from build123d import *

# Parameters (mm, degrees)
SKETCH1_W           = 120
SKETCH1_H           = 35
BOSS_EXTRUDE1_DEPTH = 40
SKETCH2_W           = 21.39
SKETCH2_H           = 30
SKETCH2_W_2         = 22
SKETCH2_W_3         = 19.56
CUT_EXTRUDE1_DEPTH  = 30
SKETCH3_W           = 21.39
SKETCH3_H           = 22.392557851
SKETCH3_W_2         = 22
SKETCH3_W_3         = 19.56
SKETCH3_H_2         = 23.276606707
CUT_EXTRUDE2_DEPTH  = 8
FILLET1_R           = 10
SKETCH4_R           = 1.25
BOSS_EXTRUDE2_DEPTH = 4
BOSS_EXTRUDE3_DEPTH = 35


with BuildPart() as part:
    # Sketch1 → Boss-Extrude1 (new body)
    with BuildSketch(Plane(origin=(0, 0, 0), x_dir=(1, 0, 0), z_dir=(0, 1, 0))):
        with Locations((18.660377358, 10.962264151)):
            Rectangle(SKETCH1_W, SKETCH1_H)
    extrude(amount=BOSS_EXTRUDE1_DEPTH)

    # Sketch2 → Cut-Extrude1 (cut)
    with BuildSketch(Plane(origin=(0, 40, 0), x_dir=(1, 0, 0), z_dir=(0, 1, 0))):
        with Locations((-28.204622642, 8.462264151)):
            Rectangle(SKETCH2_W, SKETCH2_H)
        with Locations((-4.509622642, 8.462264151)):
            Rectangle(SKETCH2_W_2, SKETCH2_H)
        with Locations((19.490377358, 8.462264151)):
            Rectangle(SKETCH2_W_2, SKETCH2_H)
        with Locations((43.490377358, 8.462264151)):
            Rectangle(SKETCH2_W_2, SKETCH2_H)
        with Locations((66.270377358, 8.462264151)):
            Rectangle(SKETCH2_W_3, SKETCH2_H)
    extrude(amount=-CUT_EXTRUDE1_DEPTH, mode=Mode.SUBTRACT)

    # Sketch3 → Cut-Extrude2 (cut)
    with BuildSketch(Plane(origin=(0, 10, 0), x_dir=(1, 0, 0), z_dir=(0, 1, 0))):
        with Locations((-28.204622642, 12.265985226)):
            Rectangle(SKETCH3_W, SKETCH3_H)
        with Locations((-4.509622642, 12.265985226)):
            Rectangle(SKETCH3_W_2, SKETCH3_H)
        with Locations((19.490377358, 12.265985226)):
            Rectangle(SKETCH3_W_2, SKETCH3_H)
        with Locations((43.490377358, 12.265985226)):
            Rectangle(SKETCH3_W_2, SKETCH3_H)
        with Locations((66.270377358, 11.823960798)):
            Rectangle(SKETCH3_W_3, SKETCH3_H_2)
    extrude(amount=-CUT_EXTRUDE2_DEPTH, mode=Mode.SUBTRACT)

    # Fillet1
    # the kernel refuses this fillet: 10 mm, written as the material it adds along each edge
    with BuildSketch(Plane(origin=(76.050377358, 2, -0.185657444), x_dir=(0, 0, -1), z_dir=(-1, 0, 0))) as fillet1_piece_1:
        with BuildLine():
            CenterArc((9.797958971, -10), FILLET1_R, 90, 78.463040967)
            Line((0, -8), (-0.195959179, -7.96))
            ThreePointArc((-0.195959179, -7.96), (-0.2, -4), (-0.2, 0))
            Line((-0.2, 0), (0, 0.2))
            Line((0, 0.2), (9.797958971, 0.2))
            Line((9.797958971, 0.2), (9.797958971, 0))
        make_face()
    extrude(amount=44.054897428)
    with BuildSketch(Plane(origin=(54.490377358, 2, -1.0697063), x_dir=(0, 1, 0), z_dir=(-1, 0, 0))) as fillet1_piece_2:
        with BuildLine():
            CenterArc((10, 9.797958971), FILLET1_R, 180, 78.463040967)
            Line((0, 9.797958971), (-0.2, 9.797958971))
            Line((-0.2, 9.797958971), (-0.2, 0))
            Line((-0.2, 0), (0, -0.2))
            ThreePointArc((0, -0.2), (4, -0.2), (7.96, -0.195959179))
            Line((7.96, -0.195959179), (8, 0))
        make_face()
    extrude(amount=46.494897428)
    with BuildSketch(Plane(origin=(54.985274786, 2, -1.0697063), x_dir=(0, 1, 0), z_dir=(-1, 0, 0))) as fillet1_piece_3:
        with BuildLine():
            CenterArc((10, 9.797958971), FILLET1_R, 180, 78.463040967)
            Line((0, 9.797958971), (-0.2, 9.797958971))
            Line((-0.2, 9.797958971), (-0.2, 0))
            Line((-0.2, 0), (0, -0.2))
            ThreePointArc((0, -0.2), (4, -0.2), (7.96, -0.195959179))
            Line((7.96, -0.195959179), (8, 0))
        make_face()
    extrude(amount=70.989794856)
    with BuildSketch(Plane(origin=(6.985274786, 2, -1.0697063), x_dir=(0, 1, 0), z_dir=(-1, 0, 0))) as fillet1_piece_4:
        with BuildLine():
            CenterArc((10, 9.797958971), FILLET1_R, 180, 78.463040967)
            Line((0, 9.797958971), (-0.2, 9.797958971))
            Line((-0.2, 9.797958971), (-0.2, 0))
            Line((-0.2, 0), (0, -0.2))
            ThreePointArc((0, -0.2), (4, -0.2), (7.96, -0.195959179))
            Line((7.96, -0.195959179), (8, 0))
        make_face()
    extrude(amount=45.884897428)
    with BuildSketch(Plane(origin=(30.985274786, 2, -1.0697063), x_dir=(0, 0, -1), z_dir=(-1, 0, 0))) as fillet1_piece_5:
        with BuildLine():
            CenterArc((9.797958971, -10), FILLET1_R, 90, 78.463040967)
            Line((0, -8), (-0.195959179, -7.96))
            ThreePointArc((-0.195959179, -7.96), (-0.2, -4), (-0.2, 0))
            Line((-0.2, 0), (0, 0.2))
            Line((0, 0.2), (9.797958971, 0.2))
            Line((9.797958971, 0.2), (9.797958971, 0))
        make_face()
    extrude(amount=70.989794856)

    # Sketch4 → Boss-Extrude2 (add)
    with BuildSketch(Plane(origin=(0, 40, 0), x_dir=(1, 0, 0), z_dir=(0, 1, 0))):
        with Locations(Location((-38.839622642, 25.962264151, 0), (0, 0, 90))):
            Circle(SKETCH4_R)
        with Locations(Location((76.160377358, 25.962264151, 0), (0, 0, 90))):
            Circle(SKETCH4_R)
    extrude(amount=BOSS_EXTRUDE2_DEPTH)

    # Sketch5 → Boss-Extrude3 (add)
    with BuildSketch(Plane.XY.offset(6.537735849)):
        Polygon((-41.339622642, 0), (-41.339622642, -20), (78.660377358, 0), align=None)
    extrude(amount=-BOSS_EXTRUDE3_DEPTH)


solid = part.part
Could you check a few things on this model? Use its own coordinates, in mm. A direction names the side the tool comes from. Give positions to 0.01 mm unless a question says otherwise; leave off trailing zeros. Order: outer loops, then holes, each group sorted by start corner. A loop starts at its lowest first (then second) coordinate and runs counter-clockwise, first axis right, second up. Notation, with made-up numbers: (38.5, -38) -> (76.5, -38) arc R21 cw to (76.5, -23) -> close; hole circle Ø8 at (38.25, -1.5). An arc over 180 degrees is marked (long way). Answer in a Markdown table with one row per item. Add a question column.
Item 1: Please list where these lines run through material, in increasing order: probe 1 along X at (y, z) = (10, -23); probe 2 along Z at (x, y) = (-25.5, 24.5); probe 3 along Z at (x, y) = (-11.5, 5.5).
Item 2: Imagine slicing it at A-A (z = -18.5). List the corners of the cut face in (x, y) for me.
Item 3: Imagine slicing it at B-B (y = 25). List the corners of the cut face in (x, z) for me, and give its area (4 significant figures).
Item 4: Imagine slicing it at C-C (y = 5.5). List the corners of the cut face in (x, z) for me.
Item 5: I'm going to push flat-ended pins straight in: P1, Ø14, axis at x = -30, z = -16, coming from the +Y side; P2, Ø6.5, axis at x = 47.5, y = 29.5, coming from the +Z side; P3, Ø2, axis at x = 6.5, z = -17, coming from the -Y side; P4, Ø10.5, axis at x = -28, y = 15, coming from the +Z side. Where does each tip first touch, or does it pass through?
Item 6: For faces 1 (the flat face through (43, 10, 3)), 2 (the flat face through (54.49, 21, -8)), which set-ups out of +Z, -Z, +X, -X, +Y, -Y let a thin tool reach every point of the face, with its end or its side?
Item 7: We'd pull the mould along Z, two halves only. Please class faces 3 (the flat face through (78.66, 20, -11)), 4 (the flat face through (18, 17, -28.462)), 5 (the cylindrical face through (66.407, 4.194, -3.734)): pulls with the +Z half, pulls with the -Z half, needs draft (parallel to the pull), parting line crosses it, or undercut.
Item 8: Imagine slicing it at D-D (x = 12.5). List the corners of the cut face in (y, z) for me.
Result:
| question | item | result |
|---|---|---|
| 1 | probe 1 | -41.34 to -38.9, -17.51 to -15.51, 6.49 to 8.49, 30.49 to 32.49, 54.49 to 56.49, 76.05 to 78.66 |
| 1 | probe 2 | -28.46 to -23.46 |
| 1 | probe 3 | -28.46 to -23.46, -3.27 to 6.54 |
| 2 | outline | (-41.34, -20) -> (78.66, 0) -> (78.66, 40) -> (76.05, 40) -> (76.05, 2) -> (56.49, 2) -> (56.49, 40) -> (54.49, 40) -> (54.49, 2) -> (32.49, 2) -> (32.49, 40) -> (30.49, 40) -> (30.49, 2) -> (8.49, 2) -> (8.49, 40) -> (6.49, 40) -> (6.49, 2) -> (-15.51, 2) -> (-15.51, 40) -> (-17.51, 40) -> (-17.51, 2) -> (-38.9, 2) -> (-38.9, 40) -> (-41.34, 40) -> close |
| 3 | outline | (-41.34, -28.46) -> (78.66, -28.46) -> (78.66, 6.54) -> (76.05, 6.54) -> (76.05, -23.46) -> (56.49, -23.46) -> (56.49, 6.54) -> (54.49, 6.54) -> (54.49, -23.46) -> (32.49, -23.46) -> (32.49, 6.54) -> (30.49, 6.54) -> (30.49, -23.46) -> (8.49, -23.46) -> (8.49, 6.54) -> (6.49, 6.54) -> (6.49, -23.46) -> (-15.51, -23.46) -> (-15.51, 6.54) -> (-17.51, 6.54) -> (-17.51, -23.46) -> (-38.9, -23.46) -> (-38.9, 6.54) -> (-41.34, 6.54) -> close |
| 3 | area | 991.5 mm2 |
| 4 | outline | (-41.34, -28.46) -> (78.66, -28.46) -> (78.66, 6.54) -> (-41.34, 6.54) -> close; hole (-38.9, -23.46) -> (-17.51, -23.46) -> (-17.51, -3.27) -> (-38.9, -3.27) -> close; hole (-15.51, -23.46) -> (6.49, -23.46) -> (6.49, -3.27) -> (-15.51, -3.27) -> close; hole (8.49, -23.46) -> (30.49, -23.46) -> (30.49, -3.27) -> (8.49, -3.27) -> close; hole (32.49, -23.46) -> (54.49, -23.46) -> (54.49, -3.27) -> (32.49, -3.27) -> close; hole (56.49, -23.46) -> (76.05, -23.46) -> (76.05, -2.38) -> (56.49, -2.38) -> close |
| 5 | P1 | y = 2.18 |
| 5 | P2 | z = -23.46 |
| 5 | P3 | y = -12.19 |
| 5 | P4 | z = 6.54 |
| 6 | face 1 | +Z, +Y |
| 6 | face 2 | +Y |
| 7 | face 3 | needs draft |
| 7 | face 4 | pulls with the -Z half |
| 7 | face 5 | undercut |
| 8 | outline | (-11.03, -28.46) -> (40, -28.46) -> (40, -23.46) -> (2, -23.46) -> (2, -10.87) arc R10 cw to (10, -1.07) -> (10, 6.54) -> (-11.03, 6.54) -> close |
